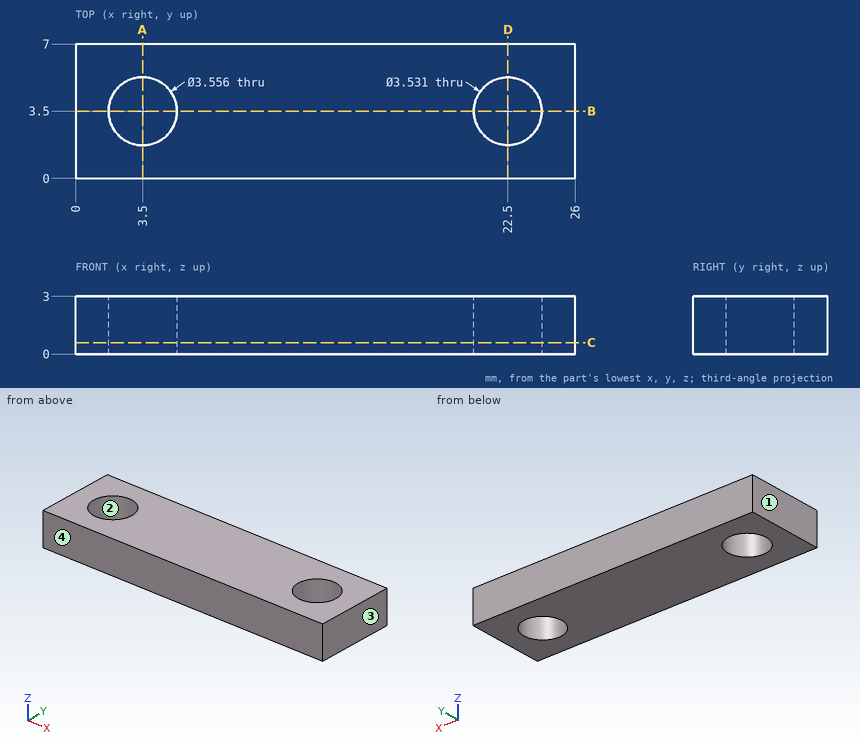
Answer from the drawing. Dimensions are ordinates in mm from the lowest x, y and z of the part. Coordinates: 2 decimals unless noted, no trailing zeros. Loops run counter-clockwise (first coordinate to the right, second up) from the corner with the lowest first, then second, coordinate; pieces in that order, holes last. Notation, with made-up numbers: (16.5, 72) - (32.5, 72) arc R28 cw to (32.5, 110) - close; hole circle Ø6 at (34, -0.5). An arc over 180 degrees is marked (long way). Use a Markdown table: item, result.
Item 1: Consider probe 1 along X at (y, z) = (3.5, 1.75) (1 decimal); probe 2 along Y at (x, z) = (22.5, 2.05) (1 decimal); probe 3 along Y at (x, z) = (21.75, 2.35). Determine where each line is inside the solid, lowest interval first. Write a range as from..to.
Evaluation:
| item | result |
|---|---|
| probe 1 | x = 0..1.7, 5.3..20.7, 24.3..26 |
| probe 2 | y = 0..1.7, 5.3..7 |
| probe 3 | y = 0..1.9, 5.1..7 |
Item 2: The mould has two halves that part along X. Classify the marked faces 1, 2, 3 and 4: +X half, -X half, draft (parallel to the pull), parting line (faces both ways), or undercut.
Evaluation:
| item | result |
|---|---|
| face 1 | -X half |
| face 2 | undercut |
| face 3 | +X half |
| face 4 | draft |
Item 3: Find section B-B, the plane y = 3.5. Determine the outline of the cut face in (x, z) (1 decimal).
Evaluation:
| item | result |
|---|---|
| outline | (0, 0) - (1.7, 0) - (1.7, 3) - (0, 3) - close; (5.3, 0) - (20.7, 0) - (20.7, 3) - (5.3, 3) - close; (24.3, 0) - (26, 0) - (26, 3) - (24.3, 3) - close |
Item 4: Given pin 1 Ø3 at (x, y) = (22.5, 3.5) entering from -Z, flat-ended and moving along its own axis, determine where the tip first touches the part or whether it passes through.
Evaluation:
| item | result |
|---|---|
| pin 1 | passes through |
Item 5: Find section A-A, the plane x = 3.5. Determine the outline of the cut face in (y, z).
Evaluation:
| item | result |
|---|---|
| outline | (0, 0) - (1.72, 0) - (1.72, 3) - (0, 3) - close; (5.28, 0) - (7, 0) - (7, 3) - (5.28, 3) - close |
Item 6: Find section D-D, the plane x = 22.5. Determine the outline of the cut face in (y, z) (1 decimal).
Evaluation:
| item | result |
|---|---|
| outline | (0, 0) - (1.7, 0) - (1.7, 3) - (0, 3) - close; (5.3, 0) - (7, 0) - (7, 3) - (5.3, 3) - close |
Item 7: Find section C-C, the plane z = 0.6. Determine the outline of the cut face in (x, y) (1 decimal), and give its area (3 significant figures).
Evaluation:
| item | result |
|---|---|
| outline | (0, 0) - (26, 0) - (26, 7) - (0, 7) - close; hole circle Ø3.6 at (3.5, 3.5); hole circle Ø3.5 at (22.5, 3.5) |
| area | 162 mm2 |
